```python
from build123d import *

# Parameters (mm, degrees)
BOSS_EXTRUDE2_DEPTH = 31
BOSS_EXTRUDE3_START = 22
BOSS_EXTRUDE3_DEPTH = 9
BOSS_EXTRUDE4_START = -22
BOSS_EXTRUDE4_DEPTH = 9
CUT_EXTRUDE3_DEPTH  = 46.022216738
CUT_EXTRUDE4_DEPTH  = 46.022216738


with BuildPart() as part:
    # Sketch2 → Boss-Extrude2 (new, symmetric)
    with BuildSketch(Plane(origin=(0, 0, 0), x_dir=(0, 0, -1), z_dir=(1, 0, 0))):
        Polygon((5, 21), (25, 21), (25, -21), (9, -21), (9, -15), (-9, -15), (-9, -21), (-25, -21), (-25, -5), (5, -5), align=None)
    extrude(amount=BOSS_EXTRUDE2_DEPTH, both=True)

    # Sketch3 → Boss-Extrude3 (add)
    with BuildSketch(Plane(origin=(0, 0, 0), x_dir=(0, 0, -1), z_dir=(1, 0, 0)).offset(BOSS_EXTRUDE3_START)):
        Polygon((5, 21), (-25, -5), (5, -5), align=None)
    extrude(amount=BOSS_EXTRUDE3_DEPTH)

    # Sketch3<4> → Boss-Extrude4 (add)
    with BuildSketch(Plane(origin=(0, 0, 0), x_dir=(0, 0, -1), z_dir=(1, 0, 0)).offset(BOSS_EXTRUDE4_START)):
        Polygon((5, 21), (-25, -5), (5, -5), align=None)
    extrude(amount=-BOSS_EXTRUDE4_DEPTH)

    # Sketch4 → Cut-Extrude3 (cut, through all)
    with BuildSketch(Plane(origin=(0, 0, 0), x_dir=(1, 0, 0), z_dir=(0, 1, 0))):
        Polygon((-9, -25), (0, -5.699437715), (9, -25), align=None)
    extrude(amount=-CUT_EXTRUDE3_DEPTH, mode=Mode.SUBTRACT)

    # Sketch6 → Cut-Extrude4 (cut, through all)
    with BuildSketch(Plane.XY):
        Polygon((-9, 21), (0, 1.699437715), (9, 21), align=None)
    extrude(amount=-CUT_EXTRUDE4_DEPTH, mode=Mode.SUBTRACT)


solid = part.part
```
For this review, take the finished solid that the model builds, in its own axes (mm). A direction names the side the tool comes from. Round coordinates to 2 decimals unless told otherwise and drop trailing zeros. Write each loop counter-clockwise with the first axis right and the second up, starting at its lowest first coordinate (ties: lowest second). Pieces come first, ordered by that corner, then holes. Notation, with made-up numbers: (-12.5, 35.25) - (-1.5, 35.25) arc R5 ccw to (-1.5, 40.25) - close; hole circle Ø11 at (20, 53.25). An arc over 180 degrees is marked (long way). Answer as a JSON object with one key per item and string values.
1. Tool access review of faces 4 (the face through (5, 8, -5)), 5 (the face through (4.437, 11.215, -14.86)), 6 (the face through (-20, 21, -15)), 7 (the face through (20, -21, 17)), 8 (the face through (0, -15, 0)): name each direction out of +Z, -Z, +X, -X, +Y, -Y from which nothing blocks a thin tool from reaching the whole face with its end or side.
Response values:
{"face 4": "+Z, +Y", "face 5": "+Z, -Z, +Y", "face 6": "+Z, -Z, +X, -X, +Y", "face 7": "+Z, -Z, +X, -X, -Y", "face 8": "+X, -X, -Y"}
2. We need section B-B on z = -16. Give the boundary of the cut face in (x, y).
Response values:
{"outline": "(-31, -21) - (31, -21) - (31, 21) - (9, 21) - (0, 1.7) - (-9, 21) - (-31, 21) - close"}
3. For pin 1 Ø4 at (x, z) = (-21.5, -4) entering from +Y, flat-tipped, find the tip position at first contact; note if it passes through.
Response values:
{"pin 1": "stops at y = 21"}
4. Draft analysis for pull direction Z (two halves, no side actions). For faces 1 (the face through (0, 0, -25)), 2 (the face through (22, 2, 4)), 3 (the face through (0, -18, -9)), state which applies: +Z half, -Z half, draft (parallel to the pull), parting line (faces both ways), or undercut.
Response values:
{"face 1": "-Z half", "face 2": "draft", "face 3": "undercut"}
5. To check wall thickness, follow line 1 along Z through (x, y) = (23, -16); line 2 along X through (y, z) = (18.5, -4); line 3 along Z through (x, y) = (-7, 5). State the ranges of each line that lie inside material, in increasing order.
Response values:
{"line 1": "z = -25 to -9, 9 to 25", "line 2": "x = -31 to -22, 22 to 31", "line 3": "z = -25 to -5"}
6. We need section C-C on y = 11.5. Give the boundary of the cut face in (x, z), then the cut area to 3 significant figures.
Response values:
{"outline": "(-31, -25) - (-4.57, -25) - (-4.57, -5) - (-22, -5) - (-22, 5.96) - (-31, 5.96) - close; (4.57, -25) - (31, -25) - (31, 5.96) - (22, 5.96) - (22, -5) - (4.57, -5) - close", "area": "1,250 mm2"}
7. We need section D-D on x = 18.5. Give the boundary of the cut face in (y, z), then the cut area to 3 significant figures.
Response values:
{"outline": "(-21, -25) - (21, -25) - (21, -5) - (-5, -5) - (-5, 25) - (-21, 25) - (-21, 9) - (-15, 9) - (-15, -9) - (-21, -9) - close", "area": "1,210 mm2"}
8. We need section A-A on y = -17.5. Give the boundary of the cut face in (x, z), then the cut area to 3 significant figures.
Response values:
{"outline": "(-31, -25) - (31, -25) - (31, -9) - (-31, -9) - close; (-31, 9) - (-1.54, 9) - (-9, 25) - (-31, 25) - close; (1.54, 9) - (31, 9) - (31, 25) - (9, 25) - close", "area": "1,820 mm2"}
